Input: part model. Units: mm. Frame: model coordinates. A direction names the side the tool comes from. Coordinates: 2 decimals unless noted, no trailing zeros. Loops run counter-clockwise (first coordinate to the right, second up) from the corner with the lowest first, then second, coordinate; pieces in that order, holes last. Notation, with made-up numbers: (-9.5, -32.5) - (48.5, -32.5) arc R24 ccw to (48.5, -10.5) - close; hole circle Ø8 at (76.25, 87). An arc over 180 degrees is marked (long way). Use a Markdown table: item, result. Add a question column.
1. Ray query, L1, parallel to X at y = 67, z = -78.5 (3 decimals); L2, parallel to Y at x = 79, z = 737 (3 decimals). Return the intervals inside material, ascending. Write a range as [from, to].
2. Section query B-B on z = 619. Return the cut outline in (x, y) (3 decimals).
3. Draft query along Z for faces 1 (the face through (1.57, -45.89, 794.13)), 2 (the face through (48, 79.375, 408)), 3 (the face through (93.685, 41.351, 360.214)). Return one class per face: released by +Z, released by -Z, zero draft, split by the parting line, or undercut.
4. Contact query for flat-ended pins moving along their axis: P1, Ø3.5, axis at x = 94, z = -43.5, coming from the +Y side; P2, Ø12, axis at x = 41.5, z = 366, coming from the -Y side (3 decimals). Output: stop coordinate, or through.
5. Section query A-A on z = -25.5. Return the cut outline in (x, y) (3 decimals).
6. Access query for faces 4 (the face through (1.57, 34.9, -116.43)), 5 (the face through (3.175, 34, 432)). Directions: +Z, -Z, +X, -X, +Y, -Y. A direction counts if a zero-diameter tool reaches every point of the face in a straight line with its end or side. Return the directions, or none.
```python
from build123d import *

# Parameters (mm, degrees)
BASE_FLANGE1_DEPTH  = 826.77
BOSS_EXTRUDE1_DEPTH = 3.175
BOSS_EXTRUDE2_START = -95.25
BOSS_EXTRUDE2_DEPTH = 3.175
BOSS_EXTRUDE3_DEPTH = 3.175
BOSS_EXTRUDE4_START = -95.25
BOSS_EXTRUDE4_DEPTH = 3.175
FILLET1_R           = 6.35
SKETCH10_R          = 2.4257
CUT_EXTRUDE1_DEPTH  = 1027.560429748
SKETCH11_R          = 4.3688
CUT_EXTRUDE2_DEPTH  = 1027.560429748
SKETCH12_R          = 17.4625
CUT_EXTRUDE3_DEPTH  = 1027.560429748
SKETCH13_R          = 3.3782
CUT_EXTRUDE4_DEPTH  = 1027.560429748
CUT_EXTRUDE5_DEPTH  = 1027.560429748
SKETCH15_R          = 4.3688
CUT_EXTRUDE6_DEPTH  = 1027.560429748
BOSS_EXTRUDE5_DEPTH = 3.175
BOSS_EXTRUDE6_START = -95.25
BOSS_EXTRUDE6_DEPTH = 3.175
SKETCH17_R          = 2.4257
CUT_EXTRUDE7_DEPTH  = 1027.560429748
FILLET3_R           = 50.8
FILLET4_R           = 6.35
SKETCH18_R          = 19.05
CUT_EXTRUDE8_DEPTH  = 1027.560429748
BOSS_EXTRUDE7_START = -3.175
SKETCH19_R          = 2.4257
BOSS_EXTRUDE7_DEPTH = 3.175
BOSS_EXTRUDE8_START = -3.175
SKETCH20_R          = 2.4257
BOSS_EXTRUDE8_DEPTH = 3.175
SKETCH21_R          = 2.4257
CUT_EXTRUDE9_DEPTH  = 1027.560429748
SKETCH22_R          = 6.35
CUT_EXTRUDE10_DEPTH = 1027.560429748
CUT_EXTRUDE11_DEPTH = 6.35
CUT_EXTRUDE12_START = -6.35
SKETCH24_W          = 28.575
SKETCH24_H          = 3.175
CUT_EXTRUDE12_DEPTH = 6.35
FILLET2_R           = 6.35


# Sheet-metal steps are written as plain solids
with BuildPart() as part:
    # Sketch1 → Base-Flange1 (new body)
    with BuildSketch(Plane.XY):
        with BuildLine():
            Line((0, 0), (0, 76.2))
            ThreePointArc((0, 76.2), (1.859871939, 80.690128061), (6.35, 82.55))
            Line((6.35, 82.55), (88.9, 82.55))
            ThreePointArc((88.9, 82.55), (93.390128061, 80.690128061), (95.25, 76.2))
            Line((95.25, 76.2), (95.25, 0))
            Line((95.25, 0), (92.075, 0))
            Line((92.075, 0), (92.075, 76.2))
            ThreePointArc((92.075, 76.2), (91.14506403, 78.44506403), (88.9, 79.375))
            Line((88.9, 79.375), (6.35, 79.375))
            ThreePointArc((6.35, 79.375), (4.10493597, 78.44506403), (3.175, 76.2))
            Line((3.175, 76.2), (3.175, 0))
            Line((3.175, 0), (0, 0))
        make_face()
    extrude(amount=BASE_FLANGE1_DEPTH)

    # Sketch8 → Boss-Extrude1 (add)
    with BuildSketch(Plane(origin=(95.25, 0, 0), x_dir=(0, 0, -1), z_dir=(1, 0, 0))):
        Polygon((-826.77, 0), (-923.757785236, 0), (-1032.58266335, 76.2), (-826.77, 76.2), align=None)
    extrude(amount=-BOSS_EXTRUDE1_DEPTH)

    # Sketch8<2> → Boss-Extrude2 (add)
    with BuildSketch(Plane(origin=(95.25, 0, 0), x_dir=(0, 0, -1), z_dir=(1, 0, 0)).offset(BOSS_EXTRUDE2_START)):
        Polygon((-826.77, 0), (-923.757785236, 0), (-1032.58266335, 76.2), (-826.77, 76.2), align=None)
    extrude(amount=BOSS_EXTRUDE2_DEPTH)

    # Sketch9 → Boss-Extrude3 (add)
    with BuildSketch(Plane(origin=(95.25, 0, 0), x_dir=(0, 0, -1), z_dir=(1, 0, 0))):
        Polygon((0, 76.2), (145.348474474, 76.2), (91.992660063, 0), (0, 0), align=None)
    extrude(amount=-BOSS_EXTRUDE3_DEPTH)

    # Sketch9<3> → Boss-Extrude4 (add)
    with BuildSketch(Plane(origin=(95.25, 0, 0), x_dir=(0, 0, -1), z_dir=(1, 0, 0)).offset(BOSS_EXTRUDE4_START)):
        Polygon((0, 76.2), (145.348474474, 76.2), (91.992660063, 0), (0, 0), align=None)
    extrude(amount=BOSS_EXTRUDE4_DEPTH)

    # Fillet1
    fillet1_edges = [part.edges().sort_by_distance(p)[0] for p in [
        (93.6625, 0, 923.757785236),
        (93.6625, 76.2, 1032.58266335),
        (1.5875, 0, 923.757785236),
        (1.5875, 76.2, 1032.58266335),
        (93.6625, 76.2, -145.348474474),
        (93.6625, 0, -91.992660063),
        (1.5875, 76.2, -145.348474474),
        (1.5875, 0, -91.992660063),
    ]]
    fillet(fillet1_edges, radius=FILLET1_R)

    # Sketch10 → Cut-Extrude1 (cut, through all)
    with BuildSketch(Plane(origin=(95.25, 0, 0), x_dir=(0, 0, -1), z_dir=(1, 0, 0))):
        with Locations(Location((102.231734197, 58.906461925, 0), (0, 0, 90))):
            Circle(SKETCH10_R)
        with Locations(Location((73.094051231, 17.293538075, 0), (0, 0, 90))):
            Circle(SKETCH10_R)
        with Locations(Location((26.031734197, 58.906461925, 0), (0, 0, 90))):
            Circle(SKETCH10_R)
        with Locations(Location((-3.105948769, 17.293538075, 0), (0, 0, 90))):
            Circle(SKETCH10_R)
        with Locations(Location((-965.096368571, 59.953262225, 0), (0, 0, 90))):
            Circle(SKETCH10_R)
        with Locations(Location((-902.676982797, 16.246737775, 0), (0, 0, 90))):
            Circle(SKETCH10_R)
        with Locations(Location((-847.621368571, 59.953262225, 0), (0, 0, 90))):
            Circle(SKETCH10_R)
        with Locations(Location((-785.201982797, 16.246737775, 0), (0, 0, 90))):
            Circle(SKETCH10_R)
    extrude(amount=-CUT_EXTRUDE1_DEPTH, mode=Mode.SUBTRACT)

    # Sketch11 → Cut-Extrude2 (cut, through all)
    with BuildSketch(Plane(origin=(0, 82.55, 0), x_dir=(1, 0, 0), z_dir=(0, 1, 0))):
        with Locations(Location((69.85, -788.67, 0), (0, 0, 270))):
            Circle(SKETCH11_R)
        with Locations(Location((69.85, -39.37, 0), (0, 0, 270))):
            Circle(SKETCH11_R)
        with Locations(Location((69.85, -388.62, 0), (0, 0, 270))):
            Circle(SKETCH11_R)
        with Locations(Location((25.4, -388.62, 0), (0, 0, 270))):
            Circle(SKETCH11_R)
        with Locations(Location((25.4, -39.37, 0), (0, 0, 270))):
            Circle(SKETCH11_R)
        with Locations(Location((25.4, -788.67, 0), (0, 0, 270))):
            Circle(SKETCH11_R)
    extrude(amount=-CUT_EXTRUDE2_DEPTH, mode=Mode.SUBTRACT)

    # Sketch12 → Cut-Extrude3 (cut, through all)
    with BuildSketch(Plane(origin=(95.25, 0, 0), x_dir=(0, 0, -1), z_dir=(1, 0, 0))):
        with Locations(Location((-342.9, 43.6245, 0), (0, 0, 90))):
            Circle(SKETCH12_R)
    extrude(amount=-CUT_EXTRUDE3_DEPTH, mode=Mode.SUBTRACT)

    # Sketch13 → Cut-Extrude4 (cut, through all)
    with BuildSketch(Plane(origin=(0, 82.55, 0), x_dir=(1, 0, 0), z_dir=(0, 1, 0))):
        with Locations(Location((47.625, -342.9, 0), (0, 0, 270))):
            Circle(SKETCH13_R)
    extrude(amount=-CUT_EXTRUDE4_DEPTH, mode=Mode.SUBTRACT)

    # Sketch14 → Cut-Extrude5 (cut, through all)
    with BuildSketch(Plane(origin=(0, 82.55, 0), x_dir=(1, 0, 0), z_dir=(0, 1, 0))):
        with BuildLine():
            Line((34.925, -826.77), (60.325, -826.77))
            Line((60.325, -826.77), (60.325, -807.72))
            ThreePointArc((60.325, -807.72), (47.625, -795.02), (34.925, -807.72))
            Line((34.925, -807.72), (34.925, -826.77))
        make_face()
    extrude(amount=-CUT_EXTRUDE5_DEPTH, mode=Mode.SUBTRACT)

    # Sketch15 → Cut-Extrude6 (cut, through all)
    with BuildSketch(Plane(origin=(95.25, 0, 0), x_dir=(0, 0, -1), z_dir=(1, 0, 0))):
        with Locations(Location((-430.905434006, 41.275, 0), (0, 0, 90))):
            Circle(SKETCH15_R)
        with Locations(Location((-684.905434006, 41.275, 0), (0, 0, 90))):
            Circle(SKETCH15_R)
        with Locations(Location((-176.905434006, 41.275, 0), (0, 0, 90))):
            Circle(SKETCH15_R)
    extrude(amount=-CUT_EXTRUDE6_DEPTH, mode=Mode.SUBTRACT)

    # Sketch16 → Boss-Extrude5 (add)
    with BuildSketch(Plane.ZY):
        with BuildLine():
            Line((921.755637927, 0), (761.999236627, 0))
            Line((761.999236627, 0), (815.216169942, -76.001657238))
            Line((815.216169942, -76.001657238), (925.397848297, 1.148384519))
            ThreePointArc((925.397848297, 1.148384519), (923.665119753, 0.293897363), (921.755637927, 0))
        make_face()
    extrude(amount=-BOSS_EXTRUDE5_DEPTH)

    # Sketch16<2> → Boss-Extrude6 (add)
    with BuildSketch(Plane.ZY.offset(BOSS_EXTRUDE6_START)):
        with BuildLine():
            Line((921.755637927, 0), (761.999236627, 0))
            Line((761.999236627, 0), (815.216169942, -76.001657238))
            Line((815.216169942, -76.001657238), (925.397848297, 1.148384519))
            ThreePointArc((925.397848297, 1.148384519), (923.665119753, 0.293897363), (921.755637927, 0))
        make_face()
    extrude(amount=BOSS_EXTRUDE6_DEPTH)

    # Sketch17 → Cut-Extrude7 (cut, through all)
    with BuildSketch(Plane.ZY):
        with Locations((823.850074628, -38.948457538)):
            Circle(SKETCH17_R)
    extrude(amount=-CUT_EXTRUDE7_DEPTH, mode=Mode.SUBTRACT)

    # Fillet3
    fillet3_edges = [part.edges().sort_by_distance(p)[0] for p in [
        (1.5875, 0, 761.999236627),
        (93.6625, 0, 761.999236627),
    ]]
    fillet(fillet3_edges, radius=FILLET3_R)

    # Fillet4
    fillet4_edges = [part.edges().sort_by_distance(p)[0] for p in [
        (1.5875, -76.001657238, 815.216169942),
        (93.6625, -76.001657238, 815.216169942),
    ]]
    fillet(fillet4_edges, radius=FILLET4_R)

    # Sketch18 → Cut-Extrude8 (cut, through all)
    with BuildSketch(Plane.ZY):
        with Locations((873.857381249, 6.144529753)):
            Circle(SKETCH18_R)
    extrude(amount=-CUT_EXTRUDE8_DEPTH, mode=Mode.SUBTRACT)

    # Sketch19 → Boss-Extrude7 (add)
    with BuildSketch(Plane.ZY.offset(BOSS_EXTRUDE7_START)):
        with Locations(Location((-26.031734197, 58.906461925, 0), (0, 0, 90))):
            Circle(SKETCH19_R)
        with Locations(Location((3.105948769, 17.293538075, 0), (0, 0, 90))):
            Circle(SKETCH19_R)
        with Locations(Location((-73.094051231, 17.293538075, 0), (0, 0, 90))):
            Circle(SKETCH19_R)
        with Locations(Location((-102.231734197, 58.906461925, 0), (0, 0, 90))):
            Circle(SKETCH19_R)
    extrude(amount=BOSS_EXTRUDE7_DEPTH)

    # Sketch20 → Boss-Extrude8 (add)
    with BuildSketch(Plane(origin=(95.25, 0, 0), x_dir=(0, 0, -1), z_dir=(1, 0, 0)).offset(BOSS_EXTRUDE8_START)):
        with Locations((102.231734197, 58.906461925)):
            Circle(SKETCH20_R)
        with Locations((73.094051231, 17.293538075)):
            Circle(SKETCH20_R)
        with Locations((-3.105948769, 17.293538075)):
            Circle(SKETCH20_R)
        with Locations((26.031734197, 58.906461925)):
            Circle(SKETCH20_R)
    extrude(amount=BOSS_EXTRUDE8_DEPTH)

    # Sketch21 → Cut-Extrude9 (cut, through all)
    with BuildSketch(Plane.ZY):
        with Locations((-121.611530794, 58.906461925)):
            Circle(SKETCH21_R)
        with Locations((-92.473847827, 17.293538075)):
            Circle(SKETCH21_R)
        with Locations((-7.311530794, 58.906461925)):
            Circle(SKETCH21_R)
        with Locations((21.826152173, 17.293538075)):
            Circle(SKETCH21_R)
    extrude(amount=-CUT_EXTRUDE9_DEPTH, mode=Mode.SUBTRACT)

    # Sketch22 → Cut-Extrude10 (cut, through all)
    with BuildSketch(Plane.ZY):
        with Locations((-53.461731718, 44.610115856)):
            Circle(SKETCH22_R)
    extrude(amount=-CUT_EXTRUDE10_DEPTH, mode=Mode.SUBTRACT)

    # Sketch23 → Cut-Extrude11 (cut)
    with BuildSketch(Plane(origin=(0, 0, 0), x_dir=(-1, 0, 0), z_dir=(0, 0, -1))):
        with BuildLine():
            Line((-3.175, 76.2), (0, 76.2))
            ThreePointArc((0, 76.2), (-1.859871939, 80.690128061), (-6.35, 82.55))
            Line((-6.35, 82.55), (-88.9, 82.55))
            ThreePointArc((-88.9, 82.55), (-93.390128061, 80.690128061), (-95.25, 76.2))
            Line((-95.25, 76.2), (-92.075, 76.2))
            ThreePointArc((-92.075, 76.2), (-91.14506403, 78.44506403), (-88.9, 79.375))
            Line((-88.9, 79.375), (-6.35, 79.375))
            ThreePointArc((-6.35, 79.375), (-4.10493597, 78.44506403), (-3.175, 76.2))
        make_face()
    extrude(amount=-CUT_EXTRUDE11_DEPTH, mode=Mode.SUBTRACT)

    # Sketch24 → Cut-Extrude12 (cut)
    with BuildSketch(Plane.XY.offset(826.77).offset(CUT_EXTRUDE12_START)):
        with BuildLine():
            ThreePointArc((6.35, 79.375), (4.10493597, 78.44506403), (3.175, 76.2))
            Line((3.175, 76.2), (0, 76.2))
            ThreePointArc((0, 76.2), (1.859871939, 80.690128061), (6.35, 82.55))
            Line((6.35, 82.55), (34.925, 82.55))
            Line((34.925, 82.55), (34.925, 79.375))
            Line((34.925, 79.375), (6.35, 79.375))
        make_face()
        with Locations((74.6125, 80.9625)):
            Rectangle(SKETCH24_W, SKETCH24_H)
        with BuildLine():
            ThreePointArc((92.075, 76.2), (91.14506403, 78.44506403), (88.9, 79.375))
            Line((88.9, 79.375), (88.9, 82.55))
            ThreePointArc((88.9, 82.55), (93.390128061, 80.690128061), (95.25, 76.2))
            Line((95.25, 76.2), (92.075, 76.2))
        make_face()
    extrude(amount=CUT_EXTRUDE12_DEPTH, mode=Mode.SUBTRACT)

    # Fillet2
    fillet2_edges = [part.edges().sort_by_distance(p)[0] for p in [
        (60.325, 80.9625, 820.42),
        (34.925, 80.9625, 820.42),
    ]]
    fillet(fillet2_edges, radius=FILLET2_R)


solid = part.part
```
Resolved:
| question | item | result |
|---|---|---|
| 1 | L1 | [0, 3.175], [92.075, 95.25] |
| 1 | L2 | [79.375, 82.55] |
| 2 | outline | (0, 0) - (3.175, 0) - (3.175, 76.2) arc R3.175 cw to (6.35, 79.375) - (88.9, 79.375) arc R3.175 cw to (92.075, 76.2) - (92.075, 0) - (95.25, 0) - (95.25, 76.2) arc R6.35 ccw to (88.9, 82.55) - (6.35, 82.55) arc R6.35 ccw to (0, 76.2) - close |
| 3 | face 1 | released by -Z |
| 3 | face 2 | zero draft |
| 3 | face 3 | undercut |
| 4 | P1 | y = 76.2 |
| 4 | P2 | y = 79.375 |
| 5 | outline | (0, 0) - (3.175, 0) - (3.175, 76.2) - (0, 76.2) - close; (92.075, 0) - (95.25, 0) - (95.25, 76.2) - (92.075, 76.2) - close |
| 6 | face 4 | -Z, +X, -X, -Y |
| 6 | face 5 | +Z, -Z, -Y |
